```python
from build123d import *

# Parameters (mm, degrees)
SKETCH_1_W           = 21
SKETCH_1_H           = 24
SKETCH_1_R           = 1.5
SKETCH_1_W_2         = 12
SKETCH_1_H_2         = 12
EXTRUDE_1_DEPTH      = 39
SKETCH_6_W           = 15
SKETCH_6_H           = 15
CUT_EXTRUDE_3_DEPTH  = 20
SKETCH_8_R           = 1.5
CUT_EXTRUDE_4_DEPTH  = 51.378566871
SKETCH_9_R           = 1
CUT_EXTRUDE_5_DEPTH  = 20
SKETCH_13_R          = 1
CUT_EXTRUDE_8_DEPTH  = 38.643060449
SKETCH_14_W          = 7
SKETCH_14_H          = 24
EXTRUDE_2_DEPTH      = 4
SKETCH_15_R          = 1.5
CUT_EXTRUDE_9_DEPTH  = 51.842895276
SKETCH_16_W          = 15
SKETCH_16_H          = 10
CUT_EXTRUDE_10_DEPTH = 54.674947601
SKETCH_17_R          = 1.5
CUT_EXTRUDE_11_DEPTH = 54.674947601
FILLET_1_R           = 1
FILLET_2_R           = 2
CHAMFER_1_SIZE       = 1


with BuildPart() as part:
    # 草图1 → 凸台-拉伸1 (new body)
    with BuildSketch(Plane.XY):
        with Locations((10.5, 12)):
            Rectangle(SKETCH_1_W, SKETCH_1_H)
        with Locations((6.5, 21)):
            Circle(SKETCH_1_R, mode=Mode.SUBTRACT)
        with Locations((14.5, 21)):
            Circle(SKETCH_1_R, mode=Mode.SUBTRACT)
        with Locations((10.5, 10.5)):
            Rectangle(SKETCH_1_W_2, SKETCH_1_H_2, mode=Mode.SUBTRACT)
    extrude(amount=EXTRUDE_1_DEPTH)

    # 草图6 → 切除-拉伸3 (cut)
    with BuildSketch(Plane(origin=(0, 0, 0), x_dir=(-1, 0, 0), z_dir=(0, 0, -1))):
        with Locations((-10.5, 10.5)):
            Rectangle(SKETCH_6_W, SKETCH_6_H)
    extrude(amount=-CUT_EXTRUDE_3_DEPTH, mode=Mode.SUBTRACT)

    # 草图8 → 切除-拉伸4 (cut, through all)
    with BuildSketch(Plane.XZ):
        with Locations(Location((10.5, 32, 0), (0, 0, 270))):
            Circle(SKETCH_8_R)
        with Locations(Location((10.5, 24, 0), (0, 0, 270))):
            Circle(SKETCH_8_R)
    extrude(amount=-CUT_EXTRUDE_4_DEPTH, mode=Mode.SUBTRACT)

    # 草图9 → 切除-拉伸5 (cut)
    with BuildSketch(Plane(origin=(0, 0, 0), x_dir=(-1, 0, 0), z_dir=(0, 0, -1))):
        with Locations((-18, 4)):
            Circle(SKETCH_9_R)
        with Locations((-18, 17)):
            Circle(SKETCH_9_R)
        with Locations((-3, 4)):
            Circle(SKETCH_9_R)
        with Locations((-3, 17)):
            Circle(SKETCH_9_R)
    extrude(amount=-CUT_EXTRUDE_5_DEPTH, mode=Mode.SUBTRACT)

    # 草图13 → 切除-拉伸8 (cut, through all)
    with BuildSketch(Plane(origin=(0, 0, 20), x_dir=(-1, 0, 0), z_dir=(0, 0, -1))):
        with Locations((-16.5, 16.5)):
            Circle(SKETCH_13_R)
        with Locations((-16.5, 4.5)):
            Circle(SKETCH_13_R)
        with Locations((-4.5, 4.5)):
            Circle(SKETCH_13_R)
        with Locations((-4.5, 16.5)):
            Circle(SKETCH_13_R)
    extrude(amount=-CUT_EXTRUDE_8_DEPTH, mode=Mode.SUBTRACT)

    # 草图14 → 凸台-拉伸2 (add)
    with BuildSketch(Plane.XY.offset(39)):
        with Locations((-3.5, 12)):
            Rectangle(SKETCH_14_W, SKETCH_14_H)
        with Locations((24.5, 12)):
            Rectangle(SKETCH_14_W, SKETCH_14_H)
    extrude(amount=-EXTRUDE_2_DEPTH)

    # 草图15 → 切除-拉伸9 (cut, through all)
    with BuildSketch(Plane(origin=(0, 0, 35), x_dir=(-1, 0, 0), z_dir=(0, 0, -1))):
        with Locations((3.5, 5)):
            Circle(SKETCH_15_R)
        with Locations((3.5, 19)):
            Circle(SKETCH_15_R)
        with Locations((-24.5, 5)):
            Circle(SKETCH_15_R)
        with Locations((-24.5, 19)):
            Circle(SKETCH_15_R)
    extrude(amount=-CUT_EXTRUDE_9_DEPTH, mode=Mode.SUBTRACT)

    # 草图16 → 切除-拉伸10 (cut, through all)
    with BuildSketch(Plane(origin=(0, 24, 0), x_dir=(1, 0, 0), z_dir=(0, 1, 0))):
        with Locations((10.5, -10)):
            Rectangle(SKETCH_16_W, SKETCH_16_H)
    extrude(amount=-CUT_EXTRUDE_10_DEPTH, mode=Mode.SUBTRACT)

    # 草图17 → 切除-拉伸11 (cut, through all)
    with BuildSketch(Plane.ZY):
        with Locations((32, 11)):
            Circle(SKETCH_17_R)
        with Locations((24, 11)):
            Circle(SKETCH_17_R)
    extrude(amount=-CUT_EXTRUDE_11_DEPTH, mode=Mode.SUBTRACT)

    # 圆角1
    fillet_1_edges = [part.edges().sort_by_distance(p)[0] for p in [
        (3, 21, 15),
        (3, 1.5, 15),
        (3, 1.5, 5),
        (3, 21, 5),
        (18, 21, 5),
        (18, 1.5, 5),
        (18, 1.5, 15),
        (18, 21, 15),
    ]]
    fillet(fillet_1_edges, radius=FILLET_1_R)

    # 圆角2
    fillet_2_edges = [part.edges().sort_by_distance(p)[0] for p in [
        (-7, 0, 37),
        (-7, 24, 37),
        (28, 24, 37),
        (28, 0, 37),
    ]]
    fillet(fillet_2_edges, radius=FILLET_2_R)

    # 倒角1
    chamfer_1_edges = [part.edges().sort_by_distance(p)[0] for p in [
        (10.5, 3, 0),
        (3, 10.5, 0),
        (18, 10.5, 0),
        (2, 4, 0),
        (19, 4, 0),
    ]]
    chamfer(chamfer_1_edges, length=CHAMFER_1_SIZE - 0.0001)  # a hair under: the kernel refuses the full size


solid = part.part
```
Input: part model. Units: mm. Frame: model coordinates. A direction names the side the tool comes from. Round coordinates to 2 decimals unless told otherwise and drop trailing zeros. Loops run counter-clockwise (first coordinate to the right, second up) from the corner with the lowest first, then second, coordinate; pieces in that order, holes last.
1) Pin query (flat end, axial travel): pin 1 (3 mm diameter, centred on x = 6.5, y = 14.5, fed in from -Z); pin 2 (1.5 mm diameter, centred on y = 12.5, z = 17, fed in from -X); pin 3 (5 mm diameter, centred on x = 14.5, y = 21, fed in from +Z); pin 4 (1.8 mm diameter, centred on y = 20.5, z = 9.5, fed in from +X). Return the tip coordinate at first contact, or that it passes through.
Ans:
pin 1: passes through
pin 2: stops at x = 0
pin 3: stops at z = 39
pin 4: stops at x = 21
2) Set-up query: faces 4 (the flat face through (-4, 12, 35)), 5 (the flat face through (10, 16.5, 29)), 6 (the cylindrical face through (2.22, 11.07, 30.5)), 7 (the flat face through (11, 4, 20)), 8 (the cylindrical face through (3.285, 20.958, 14.699)). Return all of +Z, -Z, +X, -X, +Y, -Y with unobstructed straight access to the full face (end or side cutting, diameter ignored); none if empty.
Ans:
face 4: -Z, -X, +Y, -Y
face 5: +Z, -Z
face 6: +X, -X
face 7: -Z
face 8: +Y, -Y
3) Section query B-B on x = 24.5. Return the cut outline in (y, z).
Ans:
outline: (0, 35) - (3.5, 35) - (3.5, 39) - (0, 39) - close; (6.5, 35) - (17.5, 35) - (17.5, 39) - (6.5, 39) - close; (20.5, 35) - (24, 35) - (24, 39) - (20.5, 39) - close
4) Section query D-D on x = 6.5. Count the separate pieces of the cut face and the enclosed holes in it, plus the area to 4 significant figures.
Ans:
separate pieces: 6
enclosed holes: 0
area: 230.5 mm2
5) Material intervals for line 1 (X direction, y = 15.25, z = 11.5); line 2 (X direction, y = 20, z = 24); line 3 (Y direction, x = 6, z = 1), sorted ascending.
Ans:
line 1: x = 0 to 3, 18 to 21
line 2: x = 0 to 5.38, 7.62 to 9, 12 to 13.38, 15.62 to 21
line 3: y = 0 to 3, 18 to 19.59, 22.41 to 24
6) Section query C-C on z = 19. Return the cut outline in (x, y), plus the area to 3 significant figures.
Ans:
outline: (0, 0) - (21, 0) - (21, 24) - (0, 24) - close; hole (3, 3) - (18, 3) arc R1 ccw to (18, 5) - (18, 16) arc R1 ccw to (18, 18) - (3, 18) arc R1 ccw to (3, 16) - (3, 5) arc R1 ccw to start; hole circle Ø3 at (6.5, 21); hole circle Ø3 at (14.5, 21)
area: 259 mm2
7) Section query A-A on y = 19. Return the cut outline in (x, z), plus the area to 3 significant figures.
Ans:
outline: (-7, 35) - (-5, 35) - (-5, 39) - (-7, 39) - close; (-2, 35) - (0, 35) - (0, 0) - (21, 0) - (21, 35) - (23, 35) - (23, 39) - (-2, 39) - close; (26, 35) - (28, 35) - (28, 39) - (26, 39) - close; hole (3, 6) arc R1 ccw to (4, 5) - (17, 5) arc R1 ccw to (18, 6) - (18, 14) arc R1 ccw to (17, 15) - (4, 15) arc R1 ccw to (3, 14) - close; hole circle Ø3 at (10.5, 24); hole circle Ø3 at (10.5, 32)
area: 688 mm2
8) Pull-direction query (X, two-part tool) for faces 1 (the flat face through (0, 12, 17)), 2 (the conical face through (1.7, 4, 0.7)), 3 (the flat face through (10, 18, 39)); classes: released by +X, released by -X, zero draft, split by the parting line, or undercut.
Ans:
face 1: released by -X
face 2: undercut
face 3: zero draft
